The figure shows three views and two pictorial views of one solid part (mm, origin at its lowest corner). Answer the questions. A direction names the side the tool comes from. Give positions to 0.01 mm unless a question says otherwise; leave off trailing zeros. Write each loop counter-clockwise with the first axis right and the second up, starting at its lowest first coordinate (ties: lowest second). Pieces come first, ordered by that corner, then holes. Notation, with made-up numbers: M 46,56.25 L 57,56.25 A29 cw 57,76.25 Z; hole C 3,56.5 d3. An arc over 180 degrees is marked long. Return JSON: item names as keys, results as strings.
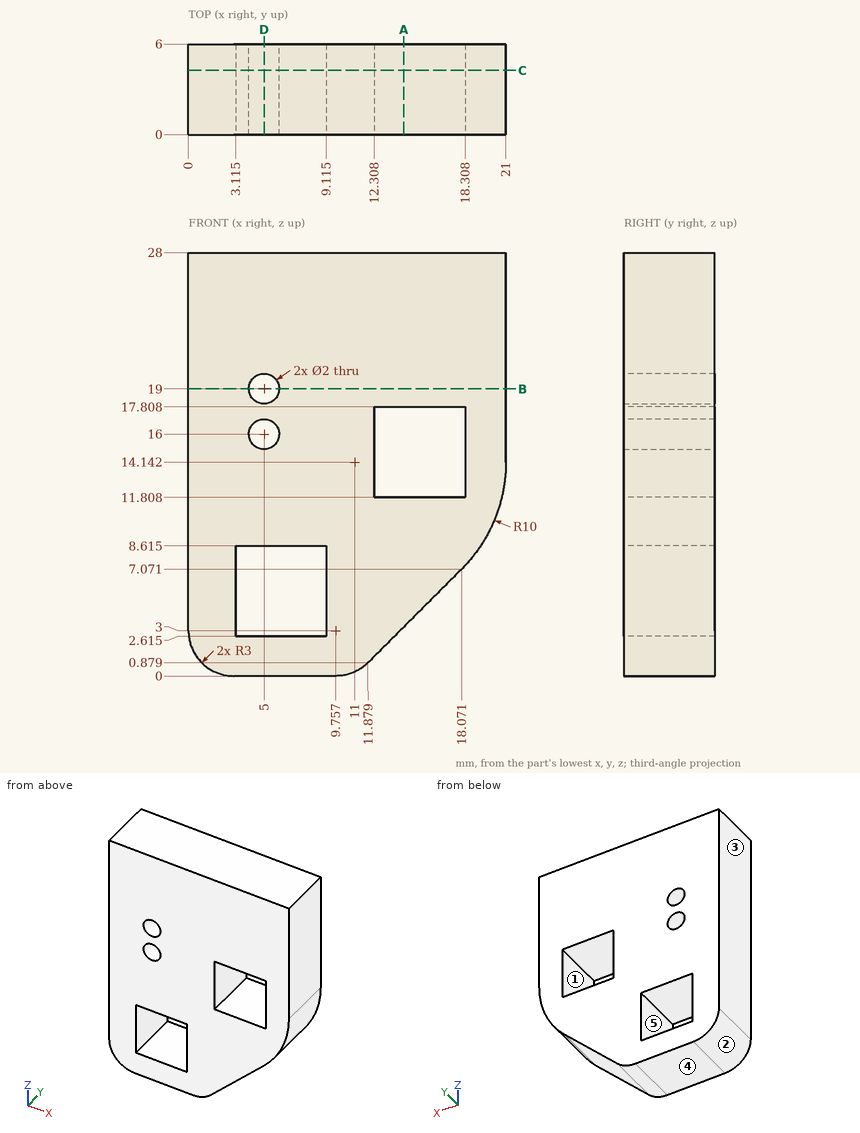
Item 1: A cutting plane is placed at C-C, the plane y = 4.25. Write down the section's boundary in (x, z) (1 decimal).
Geometry results:
{"outline": "M 0,3 A3 ccw 3,0 L 9.8,0 A3 ccw 11.9,0.9 L 18.1,7.1 A10 ccw 21,14.1 L 21,28 L 0,28 Z; hole M 3.1,2.6 L 9.1,2.6 L 9.1,8.6 L 3.1,8.6 Z; hole C 5,16 d2; hole C 5,19 d2; hole M 12.3,11.8 L 18.3,11.8 L 18.3,17.8 L 12.3,17.8 Z"}
Item 2: A cutting plane is placed at B-B, the plane z = 19. Write down the section's boundary in (x, y), plus the area to 3 significant figures.
Geometry results:
{"outline": "M 0,0 L 4,0 L 4,6 L 0,6 Z; M 6,0 L 21,0 L 21,6 L 6,6 Z", "area": "114 mm2"}
Item 3: Given pin 1 Ø3 at (y, z) = (4.5, 4.5) entering from +X; pin 2 Ø3 at (x, y) = (14.5, 1.5) entering from -Z; pin 3 Ø3 at (x, z) = (5, 16) entering from -Y, each flat-ended and moving along its own axis, determine where each tip first touches the part or whether it passes through.
Geometry results:
{"pin 1": "stops at x = 17", "pin 2": "stops at z = 2", "pin 3": "stops at y = 0"}
Item 4: A cutting plane is placed at D-D, the plane x = 5. Write down the section's boundary in (y, z) (1 decimal).
Geometry results:
{"outline": "M 0,0 L 6,0 L 6,2.6 L 0,2.6 Z; M 0,8.6 L 6,8.6 L 6,15 L 0,15 Z; M 0,17 L 6,17 L 6,18 L 0,18 Z; M 0,20 L 6,20 L 6,28 L 0,28 Z"}
Item 5: A cutting plane is placed at A-A, the plane x = 14.25. Write down the section's boundary in (y, z).
Geometry results:
{"outline": "M 0,3.25 L 6,3.25 L 6,11.81 L 0,11.81 Z; M 0,17.81 L 6,17.81 L 6,28 L 0,28 Z"}
Item 6: Determine the mould class of the marked faces 3, 4 and 5 for opening direction X: +X half, -X half, draft (parallel to the pull), parting line (faces both ways), or undercut.
Geometry results:
{"face 3": "-X half", "face 4": "draft", "face 5": "undercut"}
Item 7: Which of the six approach directions +Z, -Z, +X, -X, +Y, -Y give full straight-line access (tool end or side, diameter ignored) to the marked faces 1 and 2?
Geometry results:
{"face 1": "+Y, -Y", "face 2": "-Z, -X, +Y, -Y"}
Item 8: Find the intervals of material crossed by line 1 (X direction, y = 1.75, z = 16); line 2 (X direction, y = 1.75, z = 15.25) (1 decimal); line 3 (X direction, y = 4.75, z = 7) (1 decimal), in increasing order.
Geometry results:
{"line 1": "x = 0 to 4, 6 to 12.31, 18.31 to 21", "line 2": "x = 0 to 4.3, 5.7 to 12.3, 18.3 to 21", "line 3": "x = 0 to 3.1, 9.1 to 18"}
